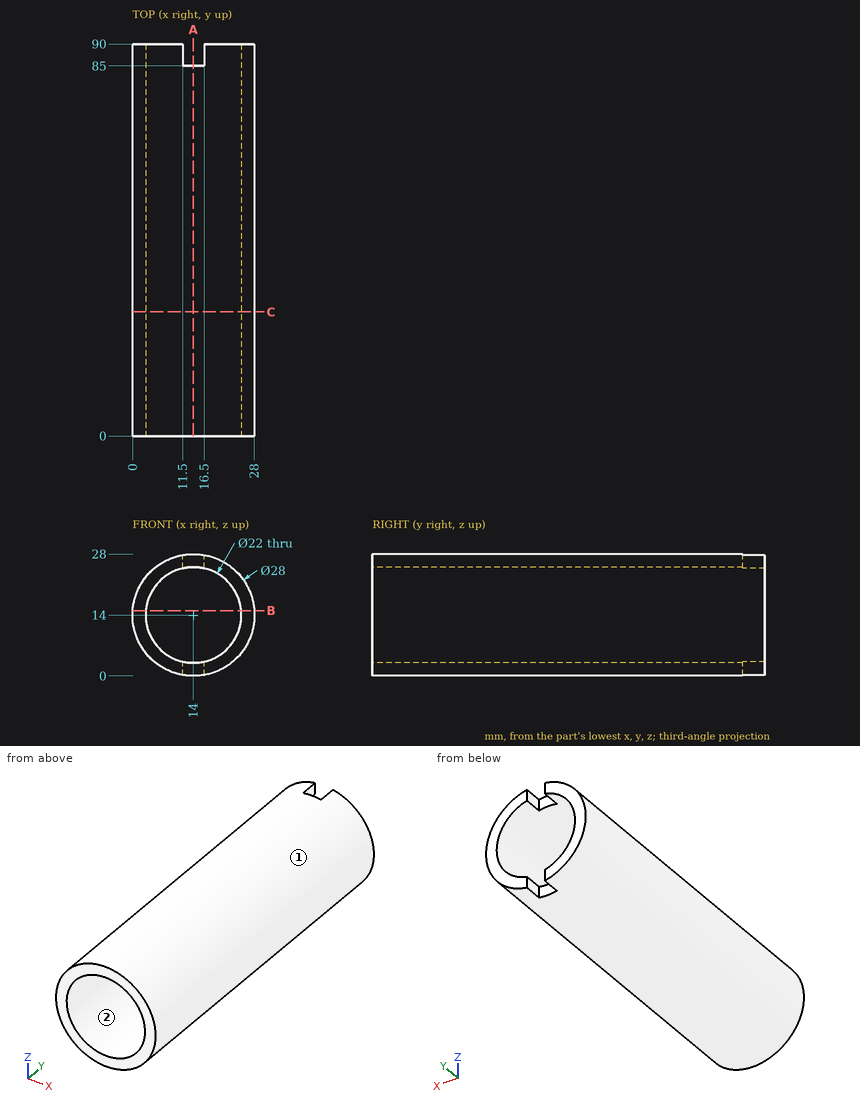
Print and shaded views of the part. All mm, measured from the part's lowest x, y and z. Coordinates: 2 decimals unless noted, no trailing zeros. Write each loop counter-clockwise with the first axis right and the second up, starting at its lowest first coordinate (ties: lowest second). Pieces come first, ordered by that corner, then holes. Notation, with made-up numbers: (55, 79) -> (82, 79) arc R29 cw to (82, 113) -> close; hole circle Ø11 at (68.25, 31.25). An arc over 180 degrees is marked (long way). Use CSV: the item, a comma, the result in double quotes. Start each with the question number.
Q1. Cut at A-A, the plane x = 14. List the corners of the cut face in (y, z), then the cut area to 3 significant figures.
Q2. Cut at C-C, the plane y = 28.5. List the corners of the cut face in (x, z).
Q3. Flat gauge pins, fed straight in: pin 1 Ø10 at (x, y) = (20, 41.5) entering from +Z; pin 2 Ø1 at (x, z) = (14, 1.5) entering from +Y; pin 3 Ø3 at (y, z) = (73, 20.5) entering from -X; pin 4 Ø3.5 at (x, z) = (13, 26) entering from +Y. Where does each tip first touch, or does it go through?
Q4. Cut at B-B, the plane z = 15. List the corners of the cut face in (x, y).
Q5. Pull direction Z, two halves, no side cores. Call the marked faces 1 and 2: released by +Z, released by -Z, zero draft, split by the parting line, or undercut.
Q6. Drill centre lines: probe 1 along X at (y, z) = (83.5, 14); probe 2 along X at (y, z) = (4.5, 17.25). Where is each one in solid material? Low to high.
Checked values:
1,outline,"(0, 0) -> (85, 0) -> (85, 3) -> (0, 3) -> close; (0, 25) -> (85, 25) -> (85, 28) -> (0, 28) -> close"
1,area,"510 mm²"
2,outline,"circle Ø28 at (14, 14); hole circle Ø22 at (14, 14)"
3,pin 1,"stops at z = 27.96"
3,pin 2,"stops at y = 85"
3,pin 3,"stops at x = 0.92"
3,pin 4,"stops at y = 90"
4,outline,"(0.04, 0) -> (3.05, 0) -> (3.05, 90) -> (0.04, 90) -> close; (24.95, 0) -> (27.96, 0) -> (27.96, 90) -> (24.95, 90) -> close"
5,face 1,"split by the parting line"
5,face 2,"undercut"
6,probe 1,"x = 0 to 3, 25 to 28"
6,probe 2,"x = 0.38 to 3.49, 24.51 to 27.62"
